```python
from build123d import *

# Parameters (mm, degrees)
F0_W     = 65
F0_H     = 50
F1_DEPTH = 2.5
F2_R     = 2.5
F3_SIZE2 = 2.49999
F3_SIZE  = 1.750509


# Not quite as in the source:
# - a fillet or chamfer is up to 0.001 mm smaller than in the source, because OpenCascade refuses the exact size


with BuildPart() as f1:
    # F0 (on Top) → F1 (new body)
    with BuildSketch(Plane.XY):
        Rectangle(F0_W, F0_H)
    extrude(amount=F1_DEPTH)

    # F2
    f2_edges = [f1.edges().sort_by_distance(p)[0] for p in [
        (-32.5, -25, 1.25),
        (32.5, -25, 1.25),
        (32.5, 25, 1.25),
        (-32.5, 25, 1.25),
    ]]
    fillet(f2_edges, radius=F2_R)

    # F3 (size 1.7505188455 and 2.5 in the source; OpenCascade refuses exactly that, so slightly less here)
    f3_edges = [f1.edges().sort_by_distance(p)[0] for p in [
        (-32.5, 0, 2.5),
        (-31.767767, 24.267767, 2.5),
        (0, 25, 2.5),
        (31.767767, 24.267767, 2.5),
        (32.5, 0, 2.5),
        (31.767767, -24.267767, 2.5),
        (0, -25, 2.5),
        (-31.767767, -24.267767, 2.5),
    ]]
    f3_side = f1.faces().sort_by_distance((0, 0, 2.5))[0]
    chamfer(f3_edges, length=F3_SIZE, length2=F3_SIZE2, reference=f3_side)


solid = f1.part
```
Geometry check sheet. Reference: the model listing, model coordinates, mm. Round coordinates to 2 decimals unless told otherwise and drop trailing zeros. Write each loop counter-clockwise with the first axis right and the second up, starting at its lowest first coordinate (ties: lowest second). Pieces come first, ordered by that corner, then holes. Notation, with made-up numbers: (8, 54.25) - (24, 54.25) arc R28 ccw to (24, 81.25) - close; hole circle Ø4 at (65.5, -13.75). An arc over 180 degrees is marked (long way). Write each question's results on one line, items separated by ' | '.
(1) Sectioned sample at A-A, the plane z = 1.8. Enter the section's corners in (x, y), plus the area to 3 significant figures.
Computed:
outline: (-31.24, -22.5) arc R1.24 ccw to (-30, -23.74) - (30, -23.74) arc R1.24 ccw to (31.24, -22.5) - (31.24, 22.5) arc R1.24 ccw to (30, 23.74) - (-30, 23.74) arc R1.24 ccw to (-31.24, 22.5) - close | area: 2,970 mm^2
(2) Thickness scan on probe 1 along Y at (x, z) = (-3, 0.2); probe 2 along X at (y, z) = (-3, 2.35); probe 3 along X at (y, z) = (-6.5, 0.95). Record the ranges inside material, lowest first. Write a range as from..to.
Computed:
probe 1: y = -24.86..24.86 | probe 2: x = -30.85..30.85 | probe 3: x = -31.83..31.83
(3) Depth check by flat-ended pin: pin 1 Ø6 at (x, y) = (-21.5, 2.5) entering from -Z. Enter the tip coordinate at first touch or a pass-through.
Computed:
pin 1: stops at z = 0
